Geometry: final body of the model. Coordinates: model frame, mm. A direction names the side the tool comes from. Round coordinates to 2 decimals unless told otherwise and drop trailing zeros. Order: outer loops, then holes, each group sorted by start corner. A loop starts at its lowest first (then second) coordinate and runs counter-clockwise, first axis right, second up. Notation, with made-up numbers: (-17, 17.5) - (-9, 17.5) arc R16 ccw to (-9, 28.5) - close; hole circle Ø7 at (46, 61). An arc over 180 degrees is marked (long way). Put each result on its own line as item: value. Start each with the question number.
(1) Material intervals for L1, parallel to Z at x = 0, y = -1.25; L2, parallel to X at y = 74, z = 1; L3, parallel to Z at x = 0, y = 64.5, sorted ascending. Write a range as [from, to].
(2) Section D-D (z = -19.05). Output: boundary loops of the cut face in (x, y), and give its area (3 significant figures).
(3) Pin query (flat end, axial travel): P1, Ø4, axis at x = -22, y = 88.5, coming from the -Z side; P2, Ø1.5, axis at y = 13.5, z = -4.5, coming from the +X side (3 decimals); P3, Ø2, axis at x = 19.5, y = 36.5, coming from the +Z side. Return the tip coordinate at first contact, or that it passes through.
(4) Section C-C (x = 19.05). Output: boundary loops of the cut face in (y, z), and give its area (3 significant figures).
(5) Section A-A (z = 0). Output: boundary loops of the cut face in (x, y), and give its area (3 significant figures).
(6) Access query for faces 1 (the face through (1, -6.35, 1)), 2 (the face through (-12.16, 50.09, 29.33)). Directions: +Z, -Z, +X, -X, +Y, -Y. A direction counts if a zero-diameter tool reaches every point of the face in a straight line with its end or side. Return the directions, or none.
(7) Section B-B (y = 76.2). Output: boundary loops of the cut face in (x, z).
(8) Pull-direction query (Y, two-part tool) for faces 3 (the face through (9.44, 79.17, 34.08)), 4 (the face through (0, 0, 0)), 5 (the face through (-0.55, -3.13, 14.87)); classes: released by +Y, released by -Y, zero draft, split by the parting line, or undercut.
from build123d import *

# Parameters (mm, degrees)
SKETCH1_R                   = 38.1
SKETCH1_R_2                 = 31.75
BOSS_EXTRUDE1_DEPTH         = 101.6
BOSS_EXTRUDE2_START         = 6.35
SKETCH2_R                   = 38.1
BOSS_EXTRUDE2_DEPTH         = 6.35
F_3_8_24_TAPPED_HOLE1_D     = 8.4328
F_3_8_24_TAPPED_HOLE1_DEPTH = 22.352
F_3_8_24_TAPPED_HOLE1_TIP   = 2.533468714
CUT_EXTRUDE1_DEPTH          = 116.003391254
CUT_EXTRUDE1_DEPTH_BACK     = 116.003391254
SKETCH8_R                   = 9.896133373


with BuildPart() as part:
    # Sketch1 → Boss-Extrude1 (new body)
    with BuildSketch(Plane(origin=(0, 0, 0), x_dir=(1, 0, 0), z_dir=(0, 1, 0))):
        with Locations(Location((0, 0, 0), (0, 0, 270))):
            Circle(SKETCH1_R)
        with Locations(Location((0, 0, 0), (0, 0, 270))):
            Circle(SKETCH1_R_2, mode=Mode.SUBTRACT)
    extrude(amount=BOSS_EXTRUDE1_DEPTH)

    # Sketch2 → Boss-Extrude2 (add)
    with BuildSketch(Plane.XZ.offset(BOSS_EXTRUDE2_START)):
        with Locations(Location((0, 0, 0), (0, 0, 270))):
            Circle(SKETCH2_R)
    extrude(amount=-BOSS_EXTRUDE2_DEPTH)

    # 3/8-24 Tapped Hole1
    with Locations(Plane(origin=(0, -6.35, 0), x_dir=(-1, 0, 0), z_dir=(0, -1, 0))):
        with Locations((0, -19.05), (19.05, 0), (0, 19.05), (-19.05, 0)):
            Hole(F_3_8_24_TAPPED_HOLE1_D / 2, depth=F_3_8_24_TAPPED_HOLE1_DEPTH)
            with Locations((0, 0, -(F_3_8_24_TAPPED_HOLE1_DEPTH + F_3_8_24_TAPPED_HOLE1_TIP / 2))):  # 118° drill point
                Cone(0, F_3_8_24_TAPPED_HOLE1_D / 2, F_3_8_24_TAPPED_HOLE1_TIP, mode=Mode.SUBTRACT)

    # Sketch8 → Cut-Extrude1 (cut, two sides: drawn at the far end of the back side and taken through both)
    with BuildSketch(Plane.XY.offset(-CUT_EXTRUDE1_DEPTH_BACK)):
        with Locations((0, 76.2)):
            Circle(SKETCH8_R)
    extrude(amount=CUT_EXTRUDE1_DEPTH + CUT_EXTRUDE1_DEPTH_BACK, mode=Mode.SUBTRACT)


solid = part.part
Checks:
1. L1: z = [-38.1, -23.27], [-14.83, 14.83], [23.27, 38.1]
1. L2: x = [-38.09, -31.73], [31.73, 38.09]
1. L3: z = [-38.1, -31.75], [31.75, 38.1]
2. outline: (-33, -6.35) - (-4.22, -6.35) - (-4.22, 0) - (-25.4, 0) - (-25.4, 101.6) - (-33, 101.6) - close; (4.22, -6.35) - (33, -6.35) - (33, 101.6) - (25.4, 101.6) - (25.4, 0) - (4.22, 0) - close
2. area: 1,910 mm²
3. P1: stops at z = -32.43
3. P2: stops at x = 37.915
3. P3: stops at z = 33.31
4. outline: (-6.35, -33) - (101.6, -33) - (101.6, -25.4) - (0, -25.4) - (0, -4.22) - (-6.35, -4.22) - close; (-6.35, 4.22) - (0, 4.22) - (0, 25.4) - (101.6, 25.4) - (101.6, 33) - (-6.35, 33) - close
4. area: 1,910 mm²
5. outline: (-38.1, -6.35) - (-23.27, -6.35) - (-23.27, 0) - (-31.75, 0) - (-31.75, 101.6) - (-38.1, 101.6) - close; (-14.83, -6.35) - (14.83, -6.35) - (14.83, 0) - (-14.83, 0) - close; (23.27, -6.35) - (38.1, -6.35) - (38.1, 101.6) - (31.75, 101.6) - (31.75, 0) - (23.27, 0) - close
5. area: 1,670 mm²
6. face 1: +Z, -Z, +X, -X, -Y
6. face 2: +Y
7. outline: (-9.9, -36.79) - (-9.9, -30.17) arc R31.75 cw to (-9.9, 30.17) - (-9.9, 36.79) arc R38.1 ccw to start; (9.9, -36.79) arc R38.1 ccw to (9.9, 36.79) - (9.9, 30.17) arc R31.75 cw to (9.9, -30.17) - close
8. face 3: undercut
8. face 4: released by +Y
8. face 5: zero draft
